Check sheet for the modelled part. Datum: model origin and axes. Units: mm. A direction names the side the tool comes from. Round coordinates to 2 decimals unless told otherwise and drop trailing zeros. Loops run counter-clockwise (first coordinate to the right, second up) from the corner with the lowest first, then second, coordinate; pieces in that order, holes last. Notation, with made-up numbers: (10, 14.5) - (17, 14.5) arc R32 ccw to (17, 47.5) - close; hole circle Ø10 at (-26, 37.5). An arc over 180 degrees is marked (long way). Put each result on its own line as item: value.
```python
from build123d import *

# Parameters (mm, degrees)
CHAMFER1_SIZE = 5


with BuildPart() as part:
    # Sketch1 → Revolve1 (revolve)
    with BuildSketch(Plane.XY, mode=Mode.PRIVATE) as revolve1_sk:
        Polygon((0, 0), (0, 62), (-10, 62), (-10, 32), (-6, 32), (-6, 0), align=None)
    revolve(revolve1_sk.sketch.rotate(Axis((0, 0, 0), (0, 1, 0)), 270), axis=Axis((0, 0, 0), (0, 1, 0)))

    # Chamfer1
    chamfer1_edges = [part.edges().sort_by_distance(p)[0] for p in [
        (0, 62, 10),
    ]]
    chamfer(chamfer1_edges, length=CHAMFER1_SIZE)

    # Sketch2 → Revolve2 (revolve)
    with BuildSketch(Plane.XY, mode=Mode.PRIVATE) as revolve2_sk:
        with BuildLine():
            Line((0, 54.5), (0, 52))
            Line((0, 52), (52.5, 52))
            ThreePointArc((52.5, 52), (46.26826484, 59.391989197), (37.928932188, 54.5))
            Line((37.928932188, 54.5), (0, 54.5))
        make_face()
    revolve(revolve2_sk.sketch.rotate(Axis((0, 52, 0), (1, 0, 0)), 90), axis=Axis((0, 52, 0), (1, 0, 0)))


solid = part.part
```
Item 1: Go/stop test with flat-tipped pins: pin 1 (12 mm diameter, centred on y = 9, z = -7, fed in from +X); pin 2 (6 mm diameter, centred on x = 30, z = 3.5, fed in from +Y); pin 3 (6 mm diameter, centred on y = 44, z = 4, fed in from -X). Record where each tip stops, or that it passes through.
Filled sheet:
pin 1: x = 5.92
pin 2: y = 54.45
pin 3: x = -9.95
Item 2: Tool access check on faces 1 (the flat face through (7, 32, 0)), 2 (the conical face through (2.035, 61.687, -4.908)). Record the directions out of +Z, -Z, +X, -X, +Y, -Y that give a thin tool (end or side, any length) a straight path to the whole face; none if there is none.
Filled sheet:
face 1: -Y
face 2: +Y
Item 3: Section check D-D on y = 28. Enter the section's corners in (x, z).
Filled sheet:
outline: circle Ø12 at (0, 0)
Item 4: Thickness scan on line 1 (X direction, y = 7, z = 0); line 2 (Y direction, x = 46.5, z = 0.5); line 3 (X direction, y = 56, z = -0.75). Record the ranges inside material, lowest first. Write a range as from..to.
Filled sheet:
line 1: -6..6
line 2: 44.67..59.33
line 3: -9.97..9.97, 38.7..51.3
Item 5: Release check for a two-part mould opening along X. For faces 3 (the cylindrical face through (23.6, 54.44, -0.54)), 4 (the cylindrical face through (-1.802, 15.776, -5.723)), 5 (the flat face through (0, 62, 0)) record: +X half, -X half, draft (parallel to the pull), parting line (faces both ways), or undercut.
Filled sheet:
face 3: undercut
face 4: parting line
face 5: draft
Item 6: Section check C-C on y = 47.5. Enter the section's corners in (x, z), then the cut area to 3 significant figures.
Filled sheet:
outline: circle Ø20 at (0, 0); circle Ø12 at (45, 0)
area: 427 mm²
Item 7: Section check B-B on z = 0. Enter the section's corners in (x, y).
Filled sheet:
outline: (-10, 32) - (-6, 32) - (-6, 0) - (6, 0) - (6, 32) - (10, 32) - (10, 49.5) - (37.93, 49.5) arc R7.5 ccw (long way) to (37.93, 54.5) - (10, 54.5) - (10, 57) - (5, 62) - (-5, 62) - (-10, 57) - close
Item 8: Section check A-A on x = 0. Enter the section's corners in (y, z), then the cut area to 3 significant figures.
Filled sheet:
outline: (0, -6) - (32, -6) - (32, -10) - (57, -10) - (62, -5) - (62, 5) - (57, 10) - (32, 10) - (32, 6) - (0, 6) - close
area: 959 mm²
